```python
from build123d import *

# Parameters (mm, degrees)
SKETCH1_R                = 120
BOSS_EXTRUDE2_DEPTH      = 100
SKETCH2_R                = 40
CUT_EXTRUDE1_DEPTH       = 100
SKETCH3_R                = 100
BOSS_EXTRUDE3_DEPTH      = 500
BOSS_EXTRUDE4_REACH      = 597.777
BOSS_EXTRUDE4_END_RADIUS = 120
SKETCH4_W                = 100
SKETCH4_H                = 105
SKETCH5_R                = 30
CUT_EXTRUDE2_DEPTH       = 40
SKETCH6_R                = 60
CUT_EXTRUDE3_DEPTH       = 40


with BuildPart() as part:
    # Sketch1 → Boss-Extrude2 (new body)
    with BuildSketch(Plane.XY):
        Circle(SKETCH1_R)
    extrude(amount=BOSS_EXTRUDE2_DEPTH)

    # Sketch2 → Cut-Extrude1 (cut)
    with BuildSketch(Plane.XY.offset(100)):
        Circle(SKETCH2_R)
    extrude(amount=-CUT_EXTRUDE1_DEPTH, mode=Mode.SUBTRACT)



with BuildPart() as body_2:
    # Sketch3 → Boss-Extrude3 (new body)
    with BuildSketch(Plane(origin=(915, 0, 0), x_dir=(0, 0, -1), z_dir=(1, 0, 0))):
        with Locations((-50, 115)):
            Circle(SKETCH3_R)
    extrude(amount=-BOSS_EXTRUDE3_DEPTH)


with BuildPart() as part_1:
    add(part.part)

    add(body_2.part)  # Boss-Extrude4 merges body 2
    # Boss-Extrude4: up to this cylinder (the profile starts outside it)
    boss_extrude4_end = Plane(origin=(0, 0, 50), z_dir=(0, 0, -1)) * Cylinder(BOSS_EXTRUDE4_END_RADIUS, 1436.554, mode=Mode.PRIVATE)
    # Sketch4 → Boss-Extrude4 (add, up to the surface)
    with BuildSketch(Plane.ZY.offset(-415), mode=Mode.PRIVATE) as boss_extrude4_sk1:
        with Locations((50, 67.5)):
            Rectangle(SKETCH4_W, SKETCH4_H)
    boss_extrude4_tool1 = extrude(boss_extrude4_sk1.sketch, amount=BOSS_EXTRUDE4_REACH, mode=Mode.PRIVATE) - boss_extrude4_end
    add(boss_extrude4_tool1.solids().sort_by_distance((415, 67.5, 50))[0])

    # Sketch5 → Cut-Extrude2 (cut)
    with BuildSketch(Plane(origin=(915, 0, 0), x_dir=(0, 0, -1), z_dir=(1, 0, 0))):
        with Locations((-50, 115)):
            Circle(SKETCH5_R)
    extrude(amount=-CUT_EXTRUDE2_DEPTH, mode=Mode.SUBTRACT)

    # Sketch6 → Cut-Extrude3 (cut)
    with BuildSketch(Plane(origin=(875, 0, 0), x_dir=(0, 0, -1), z_dir=(1, 0, 0))):
        with Locations((-50, 115)):
            Circle(SKETCH6_R)
    extrude(amount=-CUT_EXTRUDE3_DEPTH, mode=Mode.SUBTRACT)


solid = part_1.part
```
Part model, mm, in its own coordinate system. A direction names the side the tool comes from. Round coordinates to 2 decimals unless told otherwise and drop trailing zeros. Write each loop counter-clockwise with the first axis right and the second up, starting at its lowest first coordinate (ties: lowest second). Pieces come first, ordered by that corner, then holes. Notation, with made-up numbers: M 67,56 L 96,56 A24 cw 96,68 Z; hole C 76.5,-27.5 d5. An arc over 180 degrees is marked long. One line per question, with ' | ' between items.
(1) 3-axis set-ups, long thin cutter, end or side, ignore diameter. For faces 1 (the face through (92, 25, 0)), 2 (the face through (210, 120, 49)), 3 (the face through (895.28, 85.713, 56.503)), 4 (the face through (875, 143, 38)): which of +Z, -Z, +X, -X, +Y, -Y reach the whole face in a straight line?
Answer key:
face 1: -Z, -X, +Y, -Y | face 2: +Z, -Z, -X, +Y | face 3: +X | face 4: none
(2) Probe line 1 along X through (y, z) = (151.5, 91); line 2 along Y through (x, z) = (884, 50); line 3 along X through (y, z) = (66.5, 48.5). List the from-to ranges inside material, lowest first.
Answer key:
line 1: x = 415 to 835, 875 to 915 | line 2: y = 15 to 85, 145 to 215 | line 3: x = -99.89 to 835, 875 to 915
(3) Saw through at D-D on z = 129. Write the cut outline in (x, y).
Answer key:
outline: M 415,53.69 L 915,53.69 L 915,176.31 L 415,176.31 Z
(4) Saw through at A-A on y = 0. Write the cut outline in (x, z), then the cut area to 3 significant figures.
Answer key:
outline: M -120,0 L -40,0 L -40,100 L -120,100 Z; M 40,0 L 120,0 L 120,100 L 40,100 Z | area: 16,000 mm^2
(5) Two-plate mould, pull along Z, no slides. Class faces 5 (the face through (855.28, 78.491, 97.614)), 6 (the face through (-82.374, -87.261, 49.3)), 7 (the face through (835, 116, 51)), 8 (the face through (92, 25, 100)): released by +Z, released by -Z, zero draft, split by the parting line, or undercut.
Answer key:
face 5: undercut | face 6: zero draft | face 7: undercut | face 8: released by +Z
(6) Saw through at B-B on z = 30.5. Write the cut outline in (x, y).
Answer key:
outline: M 0,120 A120 ccw long 119.06,15 L 415,15 L 415,16.92 L 915,16.92 L 915,92.2 L 875,92.2 L 875,58.26 L 835,58.26 L 835,171.74 L 875,171.74 L 875,137.8 L 915,137.8 L 915,213.08 L 415,213.08 L 415,120 Z; hole C 0,0 d80
(7) Saw through at C-C on x = 509. Write the cut outline in (y, z), then the cut area to 3 significant figures.
Answer key:
outline: C 115,50 d200 | area: 31,400 mm^2
(8) Pin check, flat tips, straight feed: pin 1 (8 mm diameter, centred on y = -52.5, z = 76, fed in from +X); pin 2 (10 mm diameter, centred on x = 743.5, z = 20, fed in from +Y); pin 3 (1 mm diameter, centred on x = 201, y = 96, fed in from +Z). Stop position of each tip, or through.
Answer key:
pin 1: stops at x = 109.76 | pin 2: stops at y = 211.82 | pin 3: stops at z = 100
